Here's how the part is built. I have some questions about the finished solid (model axes, mm). A direction names the side the tool comes from. Give positions to 0.01 mm unless a question says otherwise; leave off trailing zeros. Loops run counter-clockwise (first coordinate to the right, second up) from the corner with the lowest first, then second, coordinate; pieces in that order, holes last. Notation, with made-up numbers: (77, 13.25) - (110, 13.25) arc R10 cw to (110, 24.25) - close; hole circle Ø2 at (39.25, 33.25). An arc over 180 degrees is marked (long way). Use one line per item in the form item = value.
from build123d import *

# Parameters (mm, degrees)
SKETCH_1_W          = 30
SKETCH_1_H          = 38
SKETCH_1_R          = 2.2
EXTRUDE_1_DEPTH     = 3.5
SKETCH_2_W          = 20
SKETCH_2_H          = 17
CUT_EXTRUDE_1_DEPTH = 10
FILLET_1_R          = 2


with BuildPart() as part:
    # 草图1 → 凸台-拉伸1 (new body)
    with BuildSketch(Plane.XY):
        Rectangle(SKETCH_1_W, SKETCH_1_H)
        with Locations((0, 12.5)):
            Circle(SKETCH_1_R, mode=Mode.SUBTRACT)
        with Locations((0, -12.5)):
            Circle(SKETCH_1_R, mode=Mode.SUBTRACT)
    extrude(amount=EXTRUDE_1_DEPTH)

    # 草图2 → 切除-拉伸1 (cut)
    with BuildSketch(Plane.XY.offset(3.5)):
        Rectangle(SKETCH_2_W, SKETCH_2_H)
    extrude(amount=-CUT_EXTRUDE_1_DEPTH, mode=Mode.SUBTRACT)

    # 圆角1
    fillet_1_edges = [part.edges().sort_by_distance(p)[0] for p in [
        (10, 8.5, 1.75),
        (10, -8.5, 1.75),
        (-10, -8.5, 1.75),
        (-10, 8.5, 1.75),
        (15, -19, 1.75),
        (-15, -19, 1.75),
        (-15, 19, 1.75),
        (15, 19, 1.75),
    ]]
    fillet(fillet_1_edges, radius=FILLET_1_R)


solid = part.part
(1) If we section it at A-A (x = 3.75): List the corners of the cut face in (y, z) for me.
Geometry says:
outline = (-19, 0) - (-8.5, 0) - (-8.5, 3.5) - (-19, 3.5) - close; (8.5, 0) - (19, 0) - (19, 3.5) - (8.5, 3.5) - close
(2) If we section it at D-D (x = 0): List the corners of the cut face in (y, z) for me.
Geometry says:
outline = (-19, 0) - (-14.7, 0) - (-14.7, 3.5) - (-19, 3.5) - close; (-10.3, 0) - (-8.5, 0) - (-8.5, 3.5) - (-10.3, 3.5) - close; (8.5, 0) - (10.3, 0) - (10.3, 3.5) - (8.5, 3.5) - close; (14.7, 0) - (19, 0) - (19, 3.5) - (14.7, 3.5) - close
(3) If I drill on probe 1 along Y at (x, z) = (0, 0.95); probe 2 along X at (y, z) = (3.5, 3); probe 3 along Y at (x, z) = (6.5, 2.9), over which ranges is the centre line in solid material (lowest first)?
Geometry says:
probe_1 = -19 to -14.7, -10.3 to -8.5, 8.5 to 10.3, 14.7 to 19
probe_2 = -15 to -10, 10 to 15
probe_3 = -19 to -8.5, 8.5 to 19
(4) For faces 1 (the cylindrical face through (14.4, -18.43, 1.77)), 2 (the cylindrical face through (-9.4, -7.93, 1.73)), which set-ups out of +Z, -Z, +X, -X, +Y, -Y let a thin tool reach every point of the face, with its end or its side?
Geometry says:
face_1 = +Z, -Z, +X, -Y
face_2 = +Z, -Z
(5) If we section it at B-B (y = -12.5): List the corners of the cut face in (x, z) for me, plus the area to 3 significant figures.
Geometry says:
outline = (-15, 0) - (-2.2, 0) - (-2.2, 3.5) - (-15, 3.5) - close; (2.2, 0) - (15, 0) - (15, 3.5) - (2.2, 3.5) - close
area = 89.6 mm²
(6) For P1, Ø4, axis at x = 0, y = 12.5, coming from the -Z side, with a flat end and sliding along its axis, tell me the tip position at first contact or that it passes through.
Geometry says:
P1 = through
(7) If we section it at C-C (z = 0.4): List the corners of the cut face in (x, y) for me, plus the area to 3 significant figures.
Geometry says:
outline = (-15, -17) arc R2 ccw to (-13, -19) - (13, -19) arc R2 ccw to (15, -17) - (15, 17) arc R2 ccw to (13, 19) - (-13, 19) arc R2 ccw to (-15, 17) - close; hole (-10, -6.5) arc R2 ccw to (-8, -8.5) - (8, -8.5) arc R2 ccw to (10, -6.5) - (10, 6.5) arc R2 ccw to (8, 8.5) - (-8, 8.5) arc R2 ccw to (-10, 6.5) - close; hole circle Ø4.4 at (0, -12.5); hole circle Ø4.4 at (0, 12.5)
area = 770 mm²
